For this review, take the finished solid that the model builds, in its own axes (mm). Face numbers are marked on the shaded views. A direction names the side the tool comes from. Give positions to 0.01 mm unless a question says otherwise; leave off trailing zeros. Order: outer loops, then holes, each group sorted by start corner. A loop starts at its lowest first (then second) coordinate and runs counter-clockwise, first axis right, second up. Notation, with made-up numbers: (4.25, 56.5) -> (27.25, 56.5) arc R15 cw to (27.25, 84.5) -> close; hole circle Ø9 at (1, 36). An arc over 180 degrees is marked (long way). Return JSON: item names as keys, results as strings. Group by question number.
1) Add section A-A (y = 5). Give the boundary of the cut face in (x, z).
2) Add section C-C (x = 15). Give the boundary of the cut face in (y, z).
3) Add section D-D (y = 8). Give the boundary of the cut face in (x, z), then the cut area to 3 significant figures.
4) Add section B-B (z = 0.75). Give the boundary of the cut face in (x, y), then the cut area to 3 significant figures.
5) For the marked faces 4, 5 and 6, list the 3-axis set-ups (+Z, -Z, +X, -X, +Y, -Y) from which the entire face can be reached by the end or side of a thin tool; tool diameter is ignored.
6) To check wall thickness, follow line 1 along Z through (x, y) = (0, 5); line 2 along Z through (x, y) = (1, 3.5); line 3 along Y through (x, z) = (-15, 2.15). State the ranges of each line that lie inside material, in increasing order.
7) The part is to be moulded in two halves that separate along Y. For the marked faces 1, 2 and 3, say which applies: released by +Y, released by -Y, zero draft, split by the parting line, or undercut.
8) Insertion check: P1, Ø1, axis at x = 12, y = 2, coming from the +Z side; P2, Ø4, axis at x = 0, z = -16, coming from the +Y side; P3, Ø0.8, axis at x = 16.5, z = 3.5, coming from the -Y side; P4, Ø1.8, axis at x = 15, y = 5, coming from the +Z side. Each pin has a flat end and moves straight along its axis. Give the tip position at first contact, or say it passes through.
from build123d import *

# Parameters (mm, degrees)
ESQUISSE1_W               = 40
ESQUISSE1_H               = 10
MAIN_DEPTH                = 3
ESQUISSE2_W               = 40
ESQUISSE2_H               = 2.9
MAKERBEAMRAIL_DEPTH       = 1
ESQUISSE3_R               = 1.5
MAKERBEAMHOLE_DEPTH       = 5
MAKERBEAMHOLEREPEAT_COUNT = 2
MAKERBEAMHOLEREPEAT_PITCH = 30
SKETCH3_W                 = 15
SKETCH3_H                 = 18.5
MAGNETSUPPORT_DEPTH       = 10
FILLET5_R                 = 3
SKETCH4_R                 = 6.2
MAGNETBIGHOLE_DEPTH       = 7
SKETCH5_R                 = 4
MAGNETSMALLHOLE_DEPTH     = 4
SKETCH6_R                 = 1.25
SUBMAGNETFIXHOLE_DEPTH    = 11


with BuildPart() as part:
    # Esquisse1 → Main (new body)
    with BuildSketch(Plane.XY):
        with Locations((0, 5)):
            Rectangle(ESQUISSE1_W, ESQUISSE1_H)
    extrude(amount=MAIN_DEPTH)

    # Esquisse2 → MakerBeamRail (add)
    with BuildSketch(Plane.XY.offset(3)):
        with Locations((0, 5)):
            Rectangle(ESQUISSE2_W, ESQUISSE2_H)
    extrude(amount=MAKERBEAMRAIL_DEPTH)

    # Esquisse3 → MakerBeamHole (cut, through all)
    with BuildSketch(Plane(origin=(0, 0, 0), x_dir=(-1, 0, 0), z_dir=(0, 0, -1))):
        with Locations((-15, 5)):
            Circle(ESQUISSE3_R)
    makerbeamhole = extrude(amount=-MAKERBEAMHOLE_DEPTH, mode=Mode.SUBTRACT)

    # MakerBeamHoleRepeat: MakerBeamHole ×2
    with Locations(*[(-i * MAKERBEAMHOLEREPEAT_PITCH, 0, 0) for i in range(1, MAKERBEAMHOLEREPEAT_COUNT)]):
        add(makerbeamhole, mode=Mode.SUBTRACT)

    # Sketch3 → MagnetSupport (add)
    with BuildSketch(Plane(origin=(0, 0, 0), x_dir=(1, 0, 0), z_dir=(0, 1, 0))):
        with Locations((0, 9.25)):
            Rectangle(SKETCH3_W, SKETCH3_H)
    extrude(amount=MAGNETSUPPORT_DEPTH)

    # Fillet5
    fillet5_edges = [part.edges().sort_by_distance(p)[0] for p in [
        (-7.5, 5, -18.5),
        (-7.5, 5, 0),
        (7.5, 5, 0),
        (7.5, 5, -18.5),
    ]]
    fillet(fillet5_edges, radius=FILLET5_R)

    # Sketch4 → MagnetBigHole (cut)
    with BuildSketch(Plane.XZ):
        with Locations((0, -7.5)):
            Circle(SKETCH4_R)
    extrude(amount=-MAGNETBIGHOLE_DEPTH, mode=Mode.SUBTRACT)

    # Sketch5 → MagnetSmallHole (cut, through all)
    with BuildSketch(Plane.XZ.offset(-7)):
        with Locations((0, -7.5)):
            Circle(SKETCH5_R)
    extrude(amount=-MAGNETSMALLHOLE_DEPTH, mode=Mode.SUBTRACT)

    # Sketch6 → SubMagnetFixHole (cut, through all)
    with BuildSketch(Plane(origin=(0, 10, 0), x_dir=(1, 0, 0), z_dir=(0, 1, 0))):
        with Locations((0, 16)):
            Circle(SKETCH6_R)
    extrude(amount=-SUBMAGNETFIXHOLE_DEPTH, mode=Mode.SUBTRACT)


solid = part.part
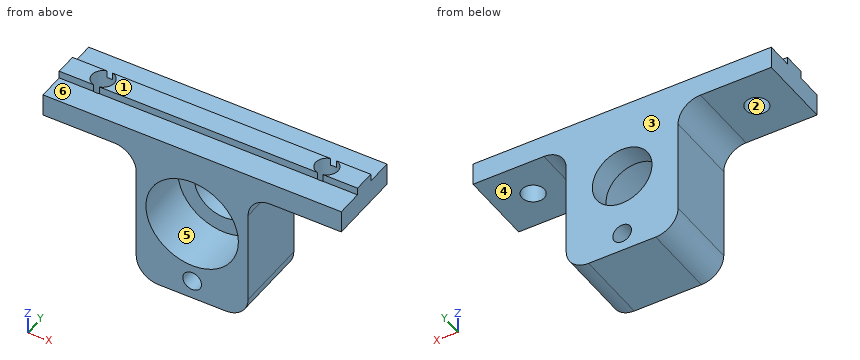
Evaluation:
{
 "1": {"outline": "(-20, 0) -> (-16.5, 0) -> (-16.5, 4) -> (-20, 4) -> close; (-13.5, 0) -> (-10.5, 0) arc R3 cw to (-7.5, -3) -> (-7.5, -15.5) arc R3 ccw to (-4.5, -18.5) -> (4.5, -18.5) arc R3 ccw to (7.5, -15.5) -> (7.5, -3) arc R3 cw to (10.5, 0) -> (13.5, 0) -> (13.5, 4) -> (-13.5, 4) -> close; (16.5, 0) -> (20, 0) -> (20, 4) -> (16.5, 4) -> close; hole circle Ø12.4 at (0, -7.5); hole circle Ø2.5 at (0, -16)"},
 "2": {"outline": "(0, 0) -> (3.5, 0) -> (3.5, 3) -> (0, 3) -> close; (6.5, 0) -> (10, 0) -> (10, 3) -> (6.5, 3) -> close"},
 "3": {"outline": "(-20, 0) -> (-10.5, 0) arc R3 cw to (-7.5, -3) -> (-7.5, -15.5) arc R3 ccw to (-4.5, -18.5) -> (4.5, -18.5) arc R3 ccw to (7.5, -15.5) -> (7.5, -3) arc R3 cw to (10.5, 0) -> (20, 0) -> (20, 3) -> (-20, 3) -> close; hole circle Ø8 at (0, -7.5); hole circle Ø2.5 at (0, -16)", "area": "342 mm^2"},
 "4": {"outline": "(-20, 0) -> (20, 0) -> (20, 10) -> (-20, 10) -> close; hole circle Ø3 at (-15, 5); hole circle Ø3 at (15, 5)", "area": "386 mm^2"},
 "5": {"face 4": "-Z, +X, +Y, -Y", "face 5": "-Y", "face 6": "+Z, +X, -X, -Y"},
 "6": {"line 1": "-18.5 to -17.25, -14.75 to -13.7, -1.3 to 4", "line 2": "-18.5 to -16.75, -15.25 to -13.62, -1.38 to 3", "line 3": "0 to 3.5, 6.5 to 10"},
 "7": {"face 1": "zero draft", "face 2": "undercut", "face 3": "released by +Y"},
 "8": {"P1": "z = 3", "P2": "y = 10", "P3": "y = 3.55", "P4": "through"}
}
